Check sheet for the modelled part. Datum: model origin and axes. Units: mm. A direction names the side the tool comes from. Round coordinates to 2 decimals unless told otherwise and drop trailing zeros. Loops run counter-clockwise (first coordinate to the right, second up) from the corner with the lowest first, then second, coordinate; pieces in that order, holes last. Notation, with made-up numbers: (49, -28.75) -> (99, -28.75) arc R26 ccw to (99, 7.25) -> close; hole circle Ø8 at (38.5, 54.5). An arc over 180 degrees is marked (long way). Return JSON: item names as keys, results as strings.
from build123d import *

# Parameters (mm, degrees)
SKETCH3_W           = 2.8
SKETCH3_H           = 0.8
SKETCH3_W_2         = 0.8
SKETCH3_H_2         = 0.1
SKETCH3_H_3         = 0.4
SKETCH3_H_4         = 6.8
SKETCH3_W_3         = 0.1
SKETCH3_W_4         = 4.65
BOSS_EXTRUDE7_DEPTH = 18
SKETCH24_W          = 6.5
SKETCH24_H          = 3
CUT_EXTRUDE25_DEPTH = 18


with BuildPart() as part:
    # Sketch3 → Boss-Extrude7 (new body)
    with BuildSketch(Plane(origin=(0, 0, 0), x_dir=(1, 0, 0), z_dir=(0, 1, 0))):
        with Locations((0, 4.5)):
            Rectangle(SKETCH3_W, SKETCH3_H)
        with Locations((0, 4.05)):
            Rectangle(SKETCH3_W_2, SKETCH3_H_2)
        with Locations((0, 3.95)):
            Rectangle(SKETCH3_W_2, SKETCH3_H_2)
        with Locations((0, 3.7)):
            Rectangle(SKETCH3_W_2, SKETCH3_H_3)
        with Locations((0, 3.45)):
            Rectangle(SKETCH3_W_2, SKETCH3_H_2)
        Rectangle(SKETCH3_W_2, SKETCH3_H_4)
        with Locations((0.45, 0)):
            Rectangle(SKETCH3_W_3, SKETCH3_H_4)
        with Locations((2.825, 0)):
            Rectangle(SKETCH3_W_4, SKETCH3_H_4)
        with Locations((-0.45, 0)):
            Rectangle(SKETCH3_W_3, SKETCH3_H_4)
        with Locations((-2.825, 0)):
            Rectangle(SKETCH3_W_4, SKETCH3_H_4)
        with Locations((0, -3.45)):
            Rectangle(SKETCH3_W_2, SKETCH3_H_2)
        with Locations((0, -3.7)):
            Rectangle(SKETCH3_W_2, SKETCH3_H_3)
        with Locations((0, -3.95)):
            Rectangle(SKETCH3_W_2, SKETCH3_H_2)
        with Locations((0, -4.05)):
            Rectangle(SKETCH3_W_2, SKETCH3_H_2)
        with Locations((0, -4.5)):
            Rectangle(SKETCH3_W, SKETCH3_H)
    extrude(amount=BOSS_EXTRUDE7_DEPTH)

    # Sketch24 → Cut-Extrude25 (cut)
    with BuildSketch(Plane(origin=(0, 18, 0), x_dir=(1, 0, 0), z_dir=(0, 1, 0))):
        Rectangle(SKETCH24_W, SKETCH24_H)
    extrude(amount=-CUT_EXTRUDE25_DEPTH, mode=Mode.SUBTRACT)


solid = part.part
Q1. Section check D-D (x = -3). Record the boundary of the cut face in (y, z).
Results list:
{"outline": "(0, -3.4) -> (18, -3.4) -> (18, -1.5) -> (0, -1.5) -> close; (0, 1.5) -> (18, 1.5) -> (18, 3.4) -> (0, 3.4) -> close"}
Q2. Go/stop test with flat-tipped pins: pin 1 (0.6 mm diameter, centred on y = 4.5, z = 4.5, fed in from +X); pin 2 (0.6 mm diameter, centred on y = 7.5, z = 4.5, fed in from -X); pin 3 (4 mm diameter, centred on x = 3.5, y = 10.5, fed in from -Z). Record where each tip stops, or that it passes through.
Results list:
{"pin 1": "x = 1.4", "pin 2": "x = -1.4", "pin 3": "z = -3.4"}
Q3. Section check B-B (x = -1). Record the boundary of the cut face in (y, z).
Results list:
{"outline": "(0, -4.9) -> (18, -4.9) -> (18, -4.1) -> (0, -4.1) -> close; (0, -3.4) -> (18, -3.4) -> (18, -1.5) -> (0, -1.5) -> close; (0, 1.5) -> (18, 1.5) -> (18, 3.4) -> (0, 3.4) -> close; (0, 4.1) -> (18, 4.1) -> (18, 4.9) -> (0, 4.9) -> close"}
Q4. Section check C-C (y = 13.25). Record the boundary of the cut face in (x, z), then the cut area to 3 significant figures.
Results list:
{"outline": "(-5.15, -3.4) -> (-0.4, -3.4) -> (-0.4, -4.1) -> (-1.4, -4.1) -> (-1.4, -4.9) -> (1.4, -4.9) -> (1.4, -4.1) -> (0.4, -4.1) -> (0.4, -3.4) -> (5.15, -3.4) -> (5.15, 3.4) -> (0.4, 3.4) -> (0.4, 4.1) -> (1.4, 4.1) -> (1.4, 4.9) -> (-1.4, 4.9) -> (-1.4, 4.1) -> (-0.4, 4.1) -> (-0.4, 3.4) -> (-5.15, 3.4) -> close; hole (-3.25, -1.5) -> (3.25, -1.5) -> (3.25, 1.5) -> (-3.25, 1.5) -> close", "area": "56.1 mm^2"}
Q5. Draft check along X on faces 1 (the flat face through (0, 9, 1.5)), 2 (the flat face through (5.15, 9, 0)), 3 (the flat face through (0, 9, 4.9)). Enter one of: released by +X, released by -X, zero draft, split by the parting line, or undercut.
Results list:
{"face 1": "undercut", "face 2": "released by +X", "face 3": "zero draft"}
Q6. Material ranges on line 1 (Z direction, x = -1.75, y = 11.75); line 2 (Z direction, x = 1, y = 4.75); line 3 (Z direction, x = 0, y = 7.75), recorded low to high.
Results list:
{"line 1": "-3.4 to -1.5, 1.5 to 3.4", "line 2": "-4.9 to -4.1, -3.4 to -1.5, 1.5 to 3.4, 4.1 to 4.9", "line 3": "-4.9 to -1.5, 1.5 to 4.9"}
Q7. Tool access check on faces 4 (the flat face through (-1, 9, 4.1)), 5 (the flat face through (1.4, 8.9, 4.5)), 6 (the flat face through (-1.4, 8.9, 4.5)). Record the directions out of +Z, -Z, +X, -X, +Y, -Y that give a thin tool (end or side, any length) a straight path to the whole face; none if there is none.
Results list:
{"face 4": "-X, +Y, -Y", "face 5": "+Z, +X, +Y, -Y", "face 6": "+Z, -X, +Y, -Y"}
Q8. Section check A-A (z = 1). Record the boundary of the cut face in (x, y), then the cut area to 3 significant figures.
Results list:
{"outline": "(-5.15, 0) -> (-3.25, 0) -> (-3.25, 18) -> (-5.15, 18) -> close; (3.25, 0) -> (5.15, 0) -> (5.15, 18) -> (3.25, 18) -> close", "area": "68.4 mm^2"}
